```python
from build123d import *

# Parameters (mm, degrees)
EXTRUDE_1_DEPTH          = 25
CUT_EXTRUDE_1_DEPTH      = 146.710678119
PATTERN_CIRCULAR_1_COUNT = 8
EXTRUDE_1_2_DEPTH        = 9.9
PATTERN_CIRCULAR_2_COUNT = 4


with BuildPart() as part:
    # Sketch 1 → Extrude 1 (new body, symmetric)
    with BuildSketch(Plane(origin=(0, 0, 0), x_dir=(1, 0, 0), z_dir=(0, 1, 0))):
        Polygon((0, -65.328148244), (46.193976626, -46.193976626), (65.328148244, 0), (46.193976626, 46.193976626), (0, 65.328148244), (-46.193976626, 46.193976626), (-65.328148244, 0), (-46.193976626, -46.193976626), align=None)
    extrude(amount=EXTRUDE_1_DEPTH, both=True)

    # Sketch 2 → Cut-Extrude 1 (cut, through all)
    with BuildSketch(Plane(origin=(55.761062435, 0, 23.096988313), x_dir=(0.382683432, 0, -0.923879533), z_dir=(0.923879533, 0, 0.382683432))):
        Polygon((-60.355339059, 25), (-60.355339059, 15), (-50.355339059, 25), align=None)
        Polygon((-60.355339059, -25), (-60.355339059, -15), (-50.355339059, -25), align=None)
    cut_extrude_1 = extrude(amount=-CUT_EXTRUDE_1_DEPTH, mode=Mode.SUBTRACT)

    # Pattern Circular 1: Cut-Extrude 1 ×8 about axis
    pattern_circular_1_axis = Axis((0, 0, 0), (0, 1, 0))
    for i in range(1, PATTERN_CIRCULAR_1_COUNT):
        add(cut_extrude_1.rotate(pattern_circular_1_axis, i * 360 / PATTERN_CIRCULAR_1_COUNT), mode=Mode.SUBTRACT)

    # Sketch 3 → Extrude 1 2 (add)
    with BuildSketch(Plane(origin=(-55.761062435, 0, -23.096988313), x_dir=(-0.382683432, 0, 0.923879533), z_dir=(-0.923879533, 0, -0.382683432))):
        Polygon((19.9, 4.565036261), (14.936812049, 10.795), (-14.936812049, 10.795), (-19.9, 4.565036261), (-19.9, -4.565036261), (-14.936812049, -10.795), (14.936812049, -10.795), (19.9, -4.565036261), align=None)
        Polygon((17.9, 3.865761475), (13.973053026, 8.795), (-13.973053026, 8.795), (-17.9, 3.865761475), (-17.9, -3.865761475), (-13.973053026, -8.795), (13.973053026, -8.795), (17.9, -3.865761475), align=None, mode=Mode.SUBTRACT)
    extrude_1_2 = extrude(amount=EXTRUDE_1_2_DEPTH)

    # Pattern Circular 2: Extrude 1 2 ×4 about axis
    pattern_circular_2_axis = Axis((0, 0, 0), (0, 1, 0))
    for i in range(1, PATTERN_CIRCULAR_2_COUNT):
        add(extrude_1_2.rotate(pattern_circular_2_axis, i * 360 / PATTERN_CIRCULAR_2_COUNT))


solid = part.part
```
Verification items for the finished model (mm, model axes). A direction names the side the tool comes from. Coordinates: 2 decimals unless noted, no trailing zeros. Loops run counter-clockwise (first coordinate to the right, second up) from the corner with the lowest first, then second, coordinate; pieces in that order, holes last. Notation, with made-up numbers: (-8.5, -29) -> (21.5, -29) arc R11 ccw to (21.5, -23) -> close; hole circle Ø7 at (61, 19). An arc over 180 degrees is marked (long way). Answer in a Markdown table with one row per item.
1) Scan lines: line 1 along Y through (x, z) = (-36, 51) (3 decimals); line 2 along Z through (x, y) = (42, 4.5); line 3 along X through (y, z) = (6, 52.5). Record each from-to range of solid material in increasing order. Write a range as from..to.
The answers:
| item | result |
|---|---|
| line 1 | y = -10.795..-8.795, 8.795..10.795 |
| line 2 | z = -55.94..-49.4, -47.93..47.93 |
| line 3 | x = -42.05..-39.28, -30.97..30.97 |
2) Section check A-A (z = 52.5). Record the cut outline in (x, y) (3 decimals), and give its area (3 significant figures).
The answers:
| item | result |
|---|---|
| outline | (-43.286, -4.565) -> (-37.914, -10.795) -> (-30.97, -10.795) -> (-30.97, -15) -> (-4.839, -25) -> (4.839, -25) -> (30.97, -15) -> (30.97, 15) -> (4.839, 25) -> (-4.839, 25) -> (-30.97, 15) -> (-30.97, 10.795) -> (-37.914, 10.795) -> (-43.286, 4.565) -> close; hole (-41.121, -3.866) -> (-36.871, -8.795) -> (-30.97, -8.795) -> (-30.97, 8.795) -> (-36.871, 8.795) -> (-41.121, 3.866) -> close |
| area | 2,650 mm2 |
3) Section check C-C (z = 33). Record the cut outline in (x, y) (3 decimals).
The answers:
| item | result |
|---|---|
| outline | (-51.659, -15) -> (-40.835, -25) -> (40.835, -25) -> (51.659, -15) -> (51.659, -10.795) -> (62.375, -10.795) -> (62.375, -8.795) -> (51.659, -8.795) -> (51.659, 8.795) -> (62.375, 8.795) -> (62.375, 10.795) -> (51.659, 10.795) -> (51.659, 15) -> (40.835, 25) -> (-40.835, 25) -> (-51.659, 15) -> close |
4) Section check D-D (y = 21). Record the cut outline in (x, z), and give its area (3 significant figures).
The answers:
| item | result |
|---|---|
| outline | (-58.83, 0) -> (-41.6, -41.6) -> (0, -58.83) -> (41.6, -41.6) -> (58.83, 0) -> (41.6, 41.6) -> (0, 58.83) -> (-41.6, 41.6) -> close |
| area | 9,790 mm2 |
5) Draft check along Y on faces 1 (the face through (-25, 10.795, 60)), 2 (the face through (-39.663, 6.365, 54.182)), 3 (the face through (-6.58, -0.06, 67.89)), 4 (the face through (-60, -10.795, -25)). Enter one of: released by +Y, released by -Y, zero draft, split by the parting line, or undercut.
The answers:
| item | result |
|---|---|
| face 1 | released by +Y |
| face 2 | undercut |
| face 3 | zero draft |
| face 4 | released by -Y |
6) Access from +Z, -Z, +X, -X, +Y, -Y to the whole of each face (thin tool, end or side, straight path). Record for faces 5 (the face through (66.949, 7.636, 8.84)), 6 (the face through (-8.9, -7.72, 66.92)), 7 (the face through (-53.591, -7.636, -41.089)).
The answers:
| item | result |
|---|---|
| face 5 | +X, +Y |
| face 6 | +Z, -Y |
| face 7 | -Z, -Y |
7) Depth check by flat-ended pin: P1, Ø22.5, axis at x = -56, z = -18, coming from the -Y side; P2, Ø4, axis at x = -10.5, y = 16.5, coming from the -Z side; P3, Ø3, axis at x = 30, y = -14.5, coming from the -Z side; P4, Ø16.5, axis at x = -17, z = 58.5, coming from the +Y side. Enter the tip coordinate at first touch or a pass-through.
The answers:
| item | result |
|---|---|
| P1 | stops at y = -25 |
| P2 | stops at z = -61.53 |
| P3 | stops at z = -53.52 |
| P4 | stops at y = 23.05 |
8) Section check B-B (y = -17.5). Record the cut outline in (x, z).
The answers:
| item | result |
|---|---|
| outline | (-62.62, 0) -> (-44.28, -44.28) -> (0, -62.62) -> (44.28, -44.28) -> (62.62, 0) -> (44.28, 44.28) -> (0, 62.62) -> (-44.28, 44.28) -> close |
